For this review, take the finished solid that the model builds, in its own axes (mm). Give positions to 0.01 mm unless a question says otherwise; leave off trailing zeros. Write each loop counter-clockwise with the first axis right and the second up, starting at its lowest first coordinate (ties: lowest second). Pieces come first, ordered by that corner, then holes.
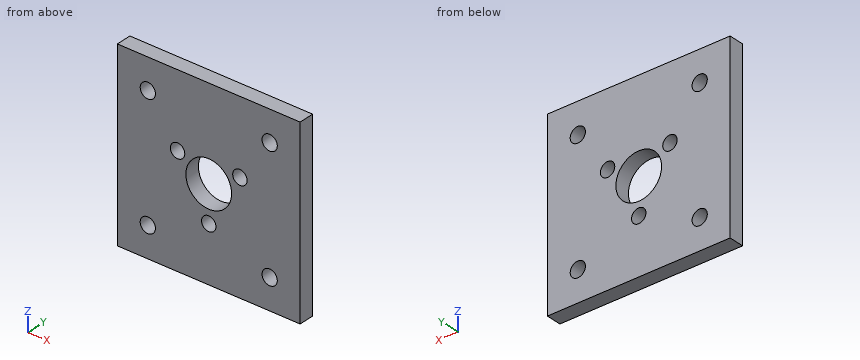
from build123d import *

# Parameters (mm, degrees)
SKETCH1_W           = 38.1
SKETCH1_H           = 38.1
BOSS_EXTRUDE1_DEPTH = 3.175
SKETCH2_R           = 1.5
SKETCH2_R_2         = 4.7625
CUT_EXTRUDE1_DEPTH  = 4.175
SKETCH3_R           = 1.5875
CUT_EXTRUDE2_DEPTH  = 4.175


with BuildPart() as part:
    # Sketch1 → Boss-Extrude1 (new body)
    with BuildSketch(Plane(origin=(0, 0, 0), x_dir=(1, 0, 0), z_dir=(0, 1, 0))):
        Rectangle(SKETCH1_W, SKETCH1_H)
    extrude(amount=BOSS_EXTRUDE1_DEPTH)

    # Sketch2 → Cut-Extrude1 (cut, through all)
    with BuildSketch(Plane(origin=(0, 3.175, 0), x_dir=(1, 0, 0), z_dir=(0, 1, 0))):
        with Locations((0, 7.5)):
            Circle(SKETCH2_R)
        with Locations((6.495190528, -3.75)):
            Circle(SKETCH2_R)
        with Locations((-6.495190528, -3.75)):
            Circle(SKETCH2_R)
        Circle(SKETCH2_R_2)
    extrude(amount=-CUT_EXTRUDE1_DEPTH, mode=Mode.SUBTRACT)

    # Sketch3 → Cut-Extrude2 (cut, through all)
    with BuildSketch(Plane(origin=(0, 3.175, 0), x_dir=(1, 0, 0), z_dir=(0, 1, 0))):
        with Locations((-12.7, 12.7)):
            Circle(SKETCH3_R)
        with Locations((-12.7, -12.7)):
            Circle(SKETCH3_R)
        with Locations((12.7, -12.7)):
            Circle(SKETCH3_R)
        with Locations((12.7, 12.7)):
            Circle(SKETCH3_R)
    extrude(amount=-CUT_EXTRUDE2_DEPTH, mode=Mode.SUBTRACT)


solid = part.part
(1) For L1, parallel to Z at x = -12.7, y = 0.8; L2, parallel to X at y = 1.6, z = 0, list the stretches that pass through material, from the lowest coordinate up.
(2) We need section A-A (x = 12.7). Count the separate pieces of the cut face and the enclosed holes in it, and give its area (3 significant figures).
(3) We need section B-B (z = -7.5). Write out the cut boundary in (x, y) (3 decimals).
(4) We need section D-D (x = -6.5). Write out the cut boundary in (y, z) (3 decimals).
(5) Clearance check with flat-ended pins moving along their axes: pin 1 Ø4 at (x, z) = (12.7, 12.7) entering from -Y; pin 2 Ø1.9 at (x, z) = (-12.7, -12.7) entering from -Y. State where each tip first meets the part, or that it passes through.
The answers:
1. L1: z = -19.05 to -14.29, -11.11 to 11.11, 14.29 to 19.05
1. L2: x = -19.05 to -4.76, 4.76 to 19.05
2. separate pieces: 3
2. enclosed holes: 0
2. area: 101 mm2
3. outline: (-19.05, 0) - (-1.5, 0) - (-1.5, 3.175) - (-19.05, 3.175) - close; (1.5, 0) - (19.05, 0) - (19.05, 3.175) - (1.5, 3.175) - close
4. outline: (0, -19.05) - (3.175, -19.05) - (3.175, 2.25) - (0, 2.25) - close; (0, 5.25) - (3.175, 5.25) - (3.175, 19.05) - (0, 19.05) - close
5. pin 1: stops at y = 0
5. pin 2: passes through
